Can you work these out from the model? Positions are in its coordinate system, mm. Give positions to 0.01 mm unless a question says otherwise; leave off trailing zeros. Order: outer loops, then holes, each group sorted by start corner. A loop starts at its lowest first (then second) coordinate and runs counter-clockwise, first axis right, second up. Notation, with made-up numbers: (-13, 51.5) - (26, 51.5) arc R9 ccw to (26, 62.5) - close; hole circle Ø1 at (-32, 74). An arc over 180 degrees is marked (long way). Return JSON: item names as keys, results as strings.
```python
from build123d import *

# Parameters (mm, degrees)
CYLINDER001_R     = 1.5
CYLINDER001_DEPTH = 10
TORUS_R           = 2
CYLINDER_R        = 15
CYLINDER_DEPTH    = 6


with BuildPart() as cilindro001:
    # Cylinder001 → Cylinder001 (new body)
    with BuildSketch(Plane.XY):
        Circle(CYLINDER001_R)
    extrude(amount=CYLINDER001_DEPTH)


with BuildPart() as toro:
    # Torus → Torus (revolve)
    with BuildSketch(Plane(origin=(0, 0, 3), x_dir=(1, 0, 0), z_dir=(0, -1, 0))):
        with Locations((15, 0)):
            Circle(TORUS_R)
    revolve(axis=Axis((0, 0, 3), (0, 0, 1)))


with BuildPart() as cut001:
    # Cylinder → Cylinder (new body)
    with BuildSketch(Plane.XY):
        Circle(CYLINDER_R)
    extrude(amount=CYLINDER_DEPTH)

    # Cut: cut Toro
    add(toro.part, mode=Mode.SUBTRACT)

    # Cut001: cut Cilindro001
    add(cilindro001.part, mode=Mode.SUBTRACT)


solid = cut001.part
```
1. Suppose I cut it at D-D (z = 1.8). List the corners of the cut face in (x, y) for me, plus the area to 3 significant figures.
Checks:
{"outline": "circle Ø26.8 at (0, 0); hole circle Ø3 at (0, 0)", "area": "557 mm^2"}
2. Suppose I cut it at A-A (y = 0). List the corners of the cut face in (x, z) for me, plus the area to 3 significant figures.
Checks:
{"outline": "(-15, 0) - (-1.5, 0) - (-1.5, 6) - (-15, 6) - (-15, 5) arc R2 cw to (-15, 1) - close; (1.5, 0) - (15, 0) - (15, 1) arc R2 cw to (15, 5) - (15, 6) - (1.5, 6) - close", "area": "149 mm^2"}
3. For pin 1 Ø6 at (x, y) = (9, 11.5) entering from -Z; pin 2 Ø3 at (y, z) = (9, 3) entering from +X; pin 3 Ø3 at (x, z) = (11, 5) entering from -Y; pin 4 Ø2.5 at (x, y) = (0, 0) entering from +Z, each with a flat end and sliding along its axis, tell me the tip position at first contact or that it passes through.
Checks:
{"pin 1": "z = 0", "pin 2": "x = 10.68", "pin 3": "y = -11.61", "pin 4": "through"}
4. Thinking about a two-plate mould opening in Y: for faces 1 (the face through (3, 0, 0)), 2 (the face through (-14.985, 0.66, 5.493)), 3 (the face through (-1.5, 0.07, 2.96)), which applies, +Y half, -Y half, draft (parallel to the pull), parting line (faces both ways), or undercut?
Checks:
{"face 1": "draft", "face 2": "parting line", "face 3": "undercut"}
5. If I drill on L1, parallel to Z at x = 9.5, y = 11.5; L2, parallel to X at y = 0, z = 4.65; L3, parallel to Y at x = 0, z = 3.75, over which ranges is the centre line in solid material (lowest first)? Write a range as [from, to].
Checks:
{"L1": "[0, 1], [5, 6]", "L2": "[-13.87, -1.5], [1.5, 13.87]", "L3": "[-13.15, -1.5], [1.5, 13.15]"}
6. Suppose I cut it at C-C (z = 5.5). List the corners of the cut face in (x, y) for me.
Checks:
{"outline": "circle Ø30 at (0, 0); hole circle Ø3 at (0, 0)"}
